The listing builds one solid part. Answer for the finished solid, in the listing's coordinates (mm). Coordinates: 2 decimals unless noted, no trailing zeros. Write each loop counter-clockwise with the first axis right and the second up, starting at its lowest first coordinate (ties: lowest second). Pieces come first, ordered by that corner, then holes. Notation, with made-up numbers: M -21.5,28.25 L 22.5,28.25 A23 ccw 22.5,66.25 Z; hole C -1,-14.75 d3. An arc over 180 degrees is marked long. Write item = value, one per line. Start each with the question number.
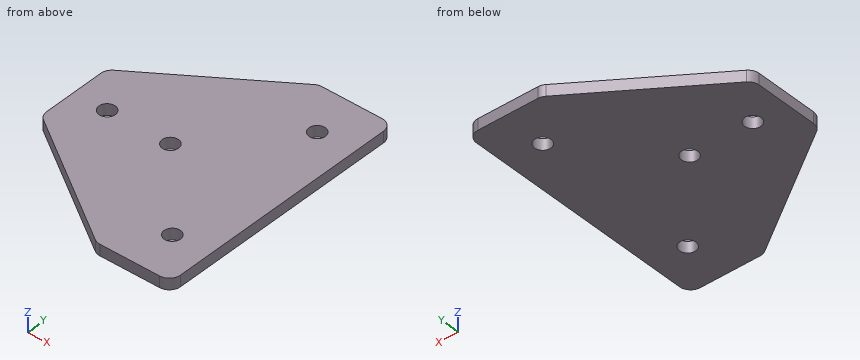
```python
from build123d import *

# Parameters (mm, degrees)
BOSS_EXTRUDE1_DEPTH = 3
SKETCH2_R           = 2.2
CUT_EXTRUDE1_DEPTH  = 66.842615379
FILLET1_R           = 3


with BuildPart() as part:
    # Sketch1 → Boss-Extrude1 (new body)
    with BuildSketch(Plane.XY):
        Polygon((0, -34.5), (0, 34.5), (-20, 34.5), (-56, 10), (-56, -10), (-20, -34.5), align=None)
    extrude(amount=BOSS_EXTRUDE1_DEPTH)

    # Sketch2 → Cut-Extrude1 (cut, through all)
    with BuildSketch(Plane.XY.offset(3)):
        with Locations((-47, 0)):
            Circle(SKETCH2_R)
        with Locations((-30, 0)):
            Circle(SKETCH2_R)
        with Locations((-10, 22.5)):
            Circle(SKETCH2_R)
        with Locations((-10, -22.5)):
            Circle(SKETCH2_R)
    extrude(amount=-CUT_EXTRUDE1_DEPTH, mode=Mode.SUBTRACT)

    # Fillet1
    fillet1_edges = [part.edges().sort_by_distance(p)[0] for p in [
        (-20, -34.5, 1.5),
        (-56, -10, 1.5),
        (-56, 10, 1.5),
        (-20, 34.5, 1.5),
        (0, 34.5, 1.5),
        (0, -34.5, 1.5),
    ]]
    fillet(fillet1_edges, radius=FILLET1_R)


solid = part.part
```
1. The part is cut by section D-D, the plane x = -30. Write down the section's boundary in (y, z).
2. Straight lines are drawn through the part: L1, parallel to Y at x = -10, z = 1; L2, parallel to X at y = 0.5, z = 0.7; L3, parallel to Y at x = -48, z = 1.65. For each, find the intervals that lie inside material, in ascending order. Write a range as [from, to].
3. The part is cut by section A-A, the plane x = -10. Write down the section's boundary in (y, z).
4. The part is cut by section B-B, the plane y = 0. Write down the section's boundary in (x, z).
5. Each of these flat-tipped pins is pushed along its axis until it touches: pin 1 (3.5 mm diameter, centred on x = -10, y = 22.5, fed in from +Z); pin 2 (1 mm diameter, centred on y = 27.5, z = 2.5, fed in from -X). Where does it stop, or does it pass through?
6. The part is cut by section C-C, the plane z = 0.8. Write down the section's boundary in (x, y), and give its area (3 significant figures).
Solution:
q1.outline = M -27.69,0 L -2.2,0 L -2.2,3 L -27.69,3 Z; M 2.2,0 L 27.69,0 L 27.69,3 L 2.2,3 Z
q2.L1 = [-34.5, -24.7], [-20.3, 20.3], [24.7, 34.5]
q2.L2 = [-56, -49.14], [-44.86, -32.14], [-27.86, 0]
q2.L3 = [-15.44, -1.96], [1.96, 15.44]
q3.outline = M -34.5,0 L -24.7,0 L -24.7,3 L -34.5,3 Z; M -20.3,0 L 20.3,0 L 20.3,3 L -20.3,3 Z; M 24.7,0 L 34.5,0 L 34.5,3 L 24.7,3 Z
q4.outline = M -56,0 L -49.2,0 L -49.2,3 L -56,3 Z; M -44.8,0 L -32.2,0 L -32.2,3 L -44.8,3 Z; M -27.8,0 L 0,0 L 0,3 L -27.8,3 Z
q5.pin_1 = through
q5.pin_2 = -31.02
q6.outline = M -56,-8.41 A3 ccw -54.69,-10.89 L -20.76,-33.98 A3 ccw -19.08,-34.5 L -3,-34.5 A3 ccw 0,-31.5 L 0,31.5 A3 ccw -3,34.5 L -19.08,34.5 A3 ccw -20.76,33.98 L -54.69,10.89 A3 ccw -56,8.41 Z; hole C -47,0 d4.4; hole C -30,0 d4.4; hole C -10,-22.5 d4.4; hole C -10,22.5 d4.4
q6.area = 2,920 mm^2
